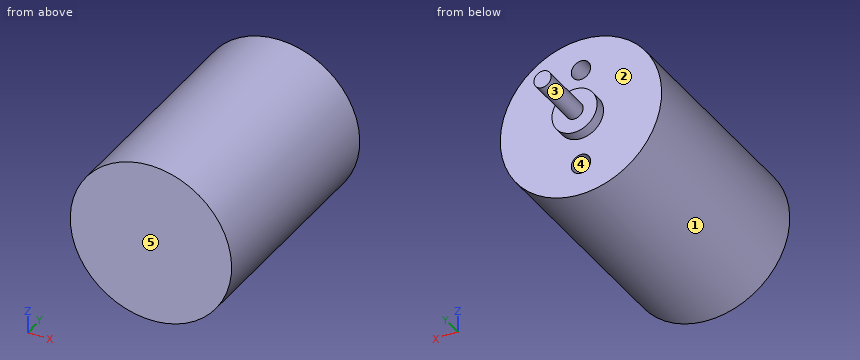
```python
from build123d import *

# Parameters (mm, degrees)
SKETCH_2_R          = 14.036295278
EXTRUDE_1_DEPTH     = 40
SKETCH_2_4_R        = 3.930162678
EXTRUDE_2_DEPTH     = 2
SKETCH_2_5_R        = 1.5
EXTRUDE_3_DEPTH     = 12
SKETCH_2_6_R        = 1.684355433
CUT_EXTRUDE_1_DEPTH = 6


with BuildPart() as part:
    # Sketch 2 → Extrude 1 (new body)
    with BuildSketch(Plane(origin=(0, 0, 0), x_dir=(1, 0, 0), z_dir=(0, 1, 0))):
        with Locations(Location((0, 0, 0), (0, 0, 270))):
            Circle(SKETCH_2_R)
    extrude(amount=-EXTRUDE_1_DEPTH)

    # Sketch 2_4 → Extrude 2 (add)
    with BuildSketch(Plane(origin=(0, 0, 0), x_dir=(1, 0, 0), z_dir=(0, 1, 0))):
        with Locations(Location((0, 0, 0), (0, 0, 270))):
            Circle(SKETCH_2_4_R)
    extrude(amount=EXTRUDE_2_DEPTH)

    # Sketch 2_5 → Extrude 3 (add)
    with BuildSketch(Plane(origin=(0, 0, 0), x_dir=(1, 0, 0), z_dir=(0, 1, 0))):
        with Locations(Location((0, 0, 0), (0, 0, 270))):
            Circle(SKETCH_2_5_R)
    extrude(amount=EXTRUDE_3_DEPTH)

    # Sketch 2_6 → Cut-Extrude 1 (cut)
    with BuildSketch(Plane(origin=(0, 0, 0), x_dir=(1, 0, 0), z_dir=(0, 1, 0))):
        with Locations(Location((0, 8.5, 0), (0, 0, 270))):
            Circle(SKETCH_2_6_R)
        with Locations(Location((0, -8.5, 0), (0, 0, 270))):
            Circle(SKETCH_2_6_R)
    extrude(amount=-CUT_EXTRUDE_1_DEPTH, mode=Mode.SUBTRACT)


solid = part.part
```
Source: CAD feature listing. Evaluate the final solid. Frame: model axes, mm. Face numbers are marked on the shaded views. A direction names the side the tool comes from. Round coordinates to 2 decimals unless told otherwise and drop trailing zeros. Loops run counter-clockwise (first coordinate to the right, second up) from the corner with the lowest first, then second, coordinate; pieces in that order, holes last. Notation, with made-up numbers: M -27.5,-19 L 21.5,-19 A24 cw 21.5,-9 Z; hole C 53,-14 d11. An arc over 180 degrees is marked long. Use a Markdown table: item, result. Add a question column.
1. Contact query for flat-ended pins moving along their axis: P1, Ø5, axis at x = 8, y = -21, coming from the -Z side; P2, Ø10, axis at x = -4.5, y = -12.5, coming from the -Z side; P3, Ø8, axis at y = -13, z = 6.5, coming from the +X side; P4, Ø5, axis at x = 10, y = -30.5, coming from the -Z side. Output: stop coordinate, or through.
2. Section query B-B on y = 5. Return the cut outline in (x, z).
3. Line query: line 1 (Y direction, x = 12.75, z = 5.5); line 2 (Y direction, x = 0.75, z = -9.5); line 3 (X direction, y = -4.1, z = -8.5). Output: solid intervals per line, ascending.
4. Mould query, pull axis Z, two halves, no side actions, for the marked faces 3, 4 and 5. Classes: pulls with the +Z half, pulls with the -Z half, needs draft (parallel to the pull), parting line crosses it, or undercut.
5. Section query D-D on z = -8.5. Return the cut outline in (x, y), then the cut area to 3 significant figures.
6. Section query C-C on x = 3. Return the cut outline in (y, z).
7. Section query A-A on z = 0. Return the cut outline in (x, y).
8. Reachability of the marked faces 1 and 2 from +Z, -Z, +X, -X, +Y, -Y: full face, straight path, thin tool, end or side. Return the list, or none.
Reported:
| question | item | result |
|---|---|---|
| 1 | P1 | stops at z = -12.91 |
| 1 | P2 | stops at z = -14.04 |
| 1 | P3 | stops at x = 13.81 |
| 1 | P4 | stops at z = -11.86 |
| 2 | outline | C 0,0 d3 |
| 3 | line 1 | y = -40 to 0 |
| 3 | line 2 | y = -40 to -6 |
| 3 | line 3 | x = -11.17 to -1.68, 1.68 to 11.17 |
| 4 | face 3 | parting line crosses it |
| 4 | face 4 | undercut |
| 4 | face 5 | needs draft |
| 5 | outline | M -11.17,-40 L 11.17,-40 L 11.17,0 L 1.68,0 L 1.68,-6 L -1.68,-6 L -1.68,0 L -11.17,0 Z |
| 5 | area | 873 mm² |
| 6 | outline | M -40,-13.71 L 0,-13.71 L 0,-2.54 L 2,-2.54 L 2,2.54 L 0,2.54 L 0,13.71 L -40,13.71 Z |
| 7 | outline | M -14.04,-40 L 14.04,-40 L 14.04,0 L 3.93,0 L 3.93,2 L 1.5,2 L 1.5,12 L -1.5,12 L -1.5,2 L -3.93,2 L -3.93,0 L -14.04,0 Z |
| 8 | face 1 | +Y, -Y |
| 8 | face 2 | +Y |
